Verification items for the finished model (mm, model axes). A direction names the side the tool comes from. Coordinates: 2 decimals unless noted, no trailing zeros. Order: outer loops, then holes, each group sorted by start corner. A loop starts at its lowest first (then second) coordinate and runs counter-clockwise, first axis right, second up. Notation, with made-up numbers: (8, 81.25) - (28, 81.25) arc R25 cw to (28, 116.25) - close; hole circle Ø2 at (10.25, 60). An arc over 180 degrees is marked (long way). Answer as CSV lines item,"result". Start each with the question number.
1. Section check C-C (z = 2.5). Record the cut outline in (x, y).
2. Material ranges on L1, parallel to Z at x = 41, y = 90; L2, parallel to X at y = -52, z = 5.5; L3, parallel to X at y = -59, z = -0.75, recorded low to high. Write a range as [from, to].
3. Section check B-B (x = 80). Record the cut outline in (y, z).
4. Set-up check for faces 5 (the cylindrical face through (84.619, -1.915, 5.986)), 6 (the cylindrical face through (-1.08, -84.88, -1.01)), 7 (the flat face through (56, -56, -2)): record each of +Z, -Z, +X, -X, +Y, -Y from which the full face is reachable in a straight line by a thin tool's end or side.
5. Go/stop test with flat-tipped pins: pin 1 (3 mm diameter, centred on y = -29, z = 3, fed in from +X); pin 2 (10 mm diameter, centred on x = 74, y = 2.5, fed in from -Z); pin 3 (1 mm diameter, centred on x = 65.5, y = -65.5, fed in from -Z); pin 4 (1.5 mm diameter, centred on y = -50, z = 1, fed in from +X). Record where each tip stops, or that it passes through.
6. Section check A-A (y = 0). Record the cut outline in (x, z).
7. Mould release check, pull along X, two halves, no side actions. Record for faces 1 (the cylindrical face through (84.619, -1.915, -1.014)), 2 (the cylindrical face through (-1.08, -84.88, 5.99)), 3 (the cylindrical face through (-53.881, -52.353, 5.986)), 4 (the flat face through (0, -80, 7)): pulls with the +X half, pulls with the -X half, needs draft (parallel to the pull), parting line crosses it, or undercut.
from build123d import *

# Parameters (mm, degrees)
SKETCH_1_R           = 100
EXTRUDE_1_DEPTH      = 5
EXTRUDE_2_DEPTH      = 2
EXTRUDE_2_DEPTH_BACK = 7
SKETCH_2_R           = 5


with BuildPart() as part:
    # Эскиз1 → Бобышка-Вытянуть1 (new body)
    with BuildSketch(Plane.XY):
        Circle(SKETCH_1_R)
    extrude(amount=EXTRUDE_1_DEPTH)

    # Эскиз2 → Бобышка-Вытянуть2 (add, two sides: drawn at the far end of the back side and taken through both)
    with BuildSketch(Plane.XY.offset(5).offset(-EXTRUDE_2_DEPTH_BACK)):
        with Locations((-80, 0)):
            Circle(SKETCH_2_R)
        with Locations((-56.568542495, -56.568542495)):
            Circle(SKETCH_2_R)
        with Locations((0, -80)):
            Circle(SKETCH_2_R)
        with Locations((56.568542495, -56.568542495)):
            Circle(SKETCH_2_R)
        with Locations((80, 0)):
            Circle(SKETCH_2_R)
    extrude(amount=EXTRUDE_2_DEPTH + EXTRUDE_2_DEPTH_BACK)


solid = part.part
Evaluation:
1,outline,"circle Ø200 at (0, 0)"
2,L1,"z = [0, 5]"
2,L2,"x = [-58.6, -54.54], [54.54, 58.6]"
2,L3,"x = [-60.94, -52.2], [52.2, 60.94]"
3,outline,"(-60, 0) - (-5, 0) - (-5, -2) - (5, -2) - (5, 0) - (60, 0) - (60, 5) - (5, 5) - (5, 7) - (-5, 7) - (-5, 5) - (-60, 5) - close"
4,face 5,"+Z"
4,face 6,"-Z"
4,face 7,"-Z, +X, -X, +Y, -Y"
5,pin 1,"stops at x = 96.14"
5,pin 2,"stops at z = -2"
5,pin 3,"stops at z = 0"
5,pin 4,"stops at x = 87.03"
6,outline,"(-100, 0) - (-85, 0) - (-85, -2) - (-75, -2) - (-75, 0) - (75, 0) - (75, -2) - (85, -2) - (85, 0) - (100, 0) - (100, 5) - (85, 5) - (85, 7) - (75, 7) - (75, 5) - (-75, 5) - (-75, 7) - (-85, 7) - (-85, 5) - (-100, 5) - close"
7,face 1,"undercut"
7,face 2,"parting line crosses it"
7,face 3,"undercut"
7,face 4,"needs draft"
